Design review of the part built by this model. Coordinates are the model's own, in mm. Face numbers are marked on the shaded views. A direction names the side the tool comes from. Give positions to 0.01 mm unless a question says otherwise; leave off trailing zeros. Loops run counter-clockwise (first coordinate to the right, second up) from the corner with the lowest first, then second, coordinate; pieces in that order, holes last. Notation, with made-up numbers: (54, 67) -> (99, 67) arc R17 ccw to (99, 96) -> close; hole circle Ø1 at (-37.75, 58.25). An arc over 180 degrees is marked (long way). Answer as CSV lines item,"result".
from build123d import *

# Parameters (mm, degrees)
ESBO_O2_W                  = 120
ESBO_O2_H                  = 120
RESSALTO_EXTRUS_O1_DEPTH   = 147.2
CORTE_EXTRUS_O1_DEPTH      = 170.905385436
CORTE_EXTRUS_O1_DEPTH_BACK = 170.905385436
ESBO_O3_W                  = 115
ESBO_O3_H                  = 115
FILETE1_R                  = 2
FILETE2_R                  = 2


with BuildPart() as part:
    # Esboço2 → Ressalto-extrusão1 (new body)
    with BuildSketch(Plane(origin=(0, 0, 0), x_dir=(1, 0, 0), z_dir=(0, 1, 0))):
        Rectangle(ESBO_O2_W, ESBO_O2_H)
    extrude(amount=RESSALTO_EXTRUS_O1_DEPTH)

    # Esboço3 → Corte-extrusão1 (cut, two sides: drawn at the far end of the back side and taken through both)
    with BuildSketch(Plane(origin=(0, 147.2, 0), x_dir=(1, 0, 0), z_dir=(0, 1, 0)).offset(-CORTE_EXTRUS_O1_DEPTH_BACK)):
        Rectangle(ESBO_O3_W, ESBO_O3_H)
    extrude(amount=CORTE_EXTRUS_O1_DEPTH + CORTE_EXTRUS_O1_DEPTH_BACK, mode=Mode.SUBTRACT)

    # Filete1
    filete1_edges = [part.edges().sort_by_distance(p)[0] for p in [
        (60, 73.6, 60),
        (-60, 73.6, 60),
        (-60, 73.6, -60),
        (60, 73.6, -60),
    ]]
    fillet(filete1_edges, radius=FILETE1_R)

    # Filete2
    filete2_edges = [part.edges().sort_by_distance(p)[0] for p in [
        (57.5, 73.6, -57.5),
        (57.5, 73.6, 57.5),
        (-57.5, 73.6, 57.5),
        (-57.5, 73.6, -57.5),
    ]]
    fillet(filete2_edges, radius=FILETE2_R)


solid = part.part
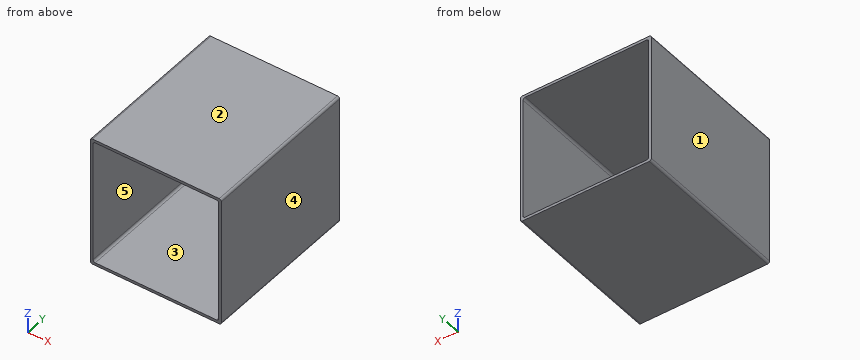
Q1. For the marked faces 4 and 5, list the 3-axis set-ups (+Z, -Z, +X, -X, +Y, -Y) from which the entire face can be reached by the end or side of a thin tool; tool diameter is ignored.
Filled sheet:
face 4,"+Z, -Z, +X, +Y, -Y"
face 5,"+Y, -Y"
Q2. To check wall thickness, follow probe 1 along X at (y, z) = (124, -32.5). State the ranges of the line that lie inside material, in increasing order. Write a range as from..to.
Filled sheet:
probe 1,"x = -60..-57.5, 57.5..60"
Q3. We need section B-B, the plane y = 40.5. State the section outline as (x, z) points, and give its area (4 significant figures).
Filled sheet:
outline,"(-60, -58) arc R2 ccw to (-58, -60) -> (58, -60) arc R2 ccw to (60, -58) -> (60, 58) arc R2 ccw to (58, 60) -> (-58, 60) arc R2 ccw to (-60, 58) -> close; hole (-57.5, -55.5) arc R2 ccw to (-55.5, -57.5) -> (55.5, -57.5) arc R2 ccw to (57.5, -55.5) -> (57.5, 55.5) arc R2 ccw to (55.5, 57.5) -> (-55.5, 57.5) arc R2 ccw to (-57.5, 55.5) -> close"
area,"1,175 mm^2"
Q4. We need section C-C, the plane x = -26. State the section outline as (y, z) points.
Filled sheet:
outline,"(0, -60) -> (147.2, -60) -> (147.2, -57.5) -> (0, -57.5) -> close; (0, 57.5) -> (147.2, 57.5) -> (147.2, 60) -> (0, 60) -> close"
Q5. We need section A-A, the plane z = -42.5. State the section outline as (x, y) points, and give its area (3 significant figures).
Filled sheet:
outline,"(-60, 0) -> (-57.5, 0) -> (-57.5, 147.2) -> (-60, 147.2) -> close; (57.5, 0) -> (60, 0) -> (60, 147.2) -> (57.5, 147.2) -> close"
area,"736 mm^2"
Q6. The part is to be moulded in two halves that separate along X. For the marked faces 1, 2 and 3, say which applies: pulls with the +X half, pulls with the -X half, needs draft (parallel to the pull), parting line crosses it, or undercut.
Filled sheet:
face 1,"pulls with the -X half"
face 2,"needs draft"
face 3,"undercut"
